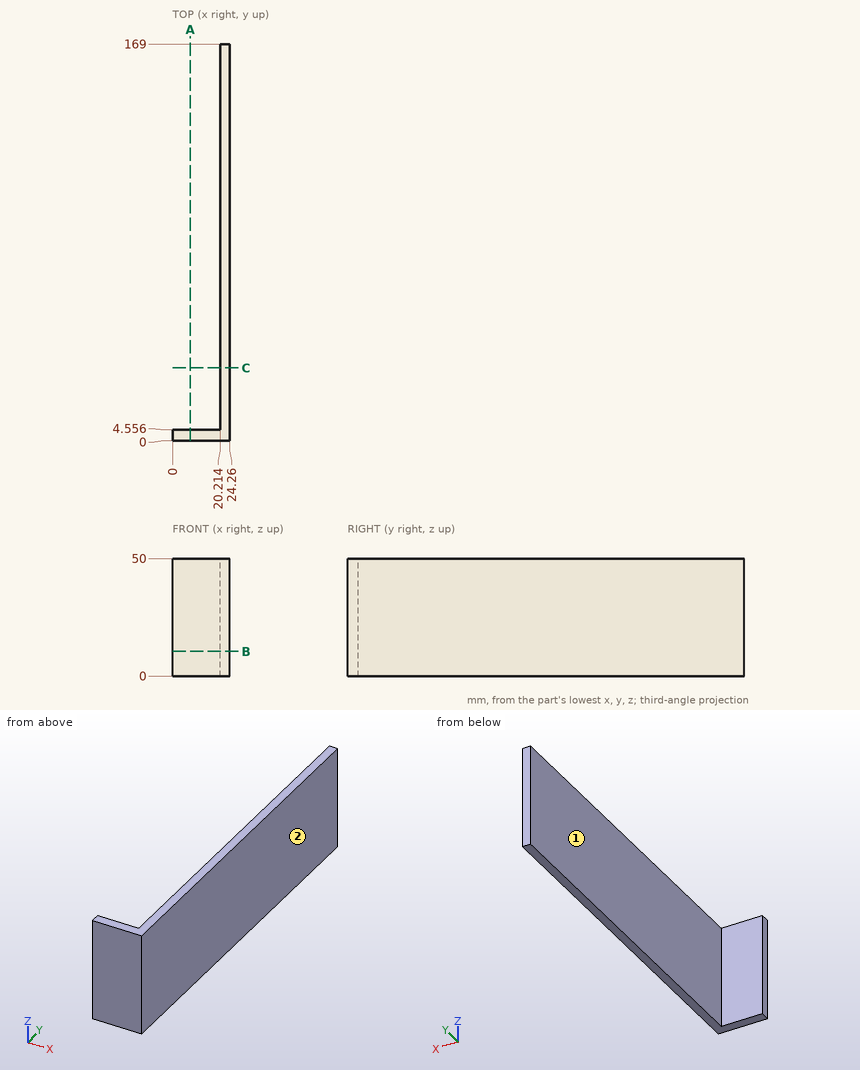
Study the drawing (mm; zero at the part's minimum x, y, z) and answer. A direction names the side the tool comes from. Coordinates: 2 decimals unless noted, no trailing zeros. Write each loop counter-clockwise with the first axis right and the second up, starting at its lowest first coordinate (ties: lowest second). Pieces come first, ordered by that corner, then holes.
Q1. A cutting plane is placed at C-C, the plane y = 31. Give the vertices of the cut face in (x, z) (1 decimal), then the cut area to 3 significant figures.
Q2. Each of these flat-tipped pins is pushed along its axis until it touches: pin 1 Ø8 at (y, z) = (61, 30.5) entering from -X; pin 2 Ø12 at (x, z) = (9, 23) entering from +Y. Where does it stop, or does it pass through?
Q3. A cutting plane is placed at B-B, the plane z = 10.5. Give the vertices of the cut face in (x, y) (1 decimal).
Q4. Which of the six approach directions +Z, -Z, +X, -X, +Y, -Y give full straight-line access (tool end or side, diameter ignored) to the marked faces 1 and 2?
Q5. Find the intervals of material crossed by line 1 (Y direction, x = 1.75, z = 41.5) (1 decimal); line 2 (X direction, y = 75.5, z = 41.5) (1 decimal), in increasing order.
Q6. A cutting plane is placed at A-A, the plane x = 7.5. Give the vertices of the cut face in (y, z) (1 decimal).
Findings below:
1. outline: (20.2, 0) - (24.3, 0) - (24.3, 50) - (20.2, 50) - close
1. area: 202 mm2
2. pin 1: stops at x = 20.21
2. pin 2: stops at y = 4.56
3. outline: (0, 0) - (24.3, 0) - (24.3, 169) - (20.2, 169) - (20.2, 4.6) - (0, 4.6) - close
4. face 1: +Z, -Z, -X, +Y
4. face 2: +Z, -Z, +X, +Y, -Y
5. line 1: y = 0 to 4.6
5. line 2: x = 20.2 to 24.3
6. outline: (0, 0) - (4.6, 0) - (4.6, 50) - (0, 50) - close
